Verification items for the finished model (mm, model axes). A direction names the side the tool comes from. Round coordinates to 2 decimals unless told otherwise and drop trailing zeros. Write each loop counter-clockwise with the first axis right and the second up, starting at its lowest first coordinate (ties: lowest second). Pieces come first, ordered by that corner, then holes. Notation, with made-up numbers: M 42.5,1 L 100.5,1 A30 ccw 100.5,36 Z; hole C 81.25,68.25 d9. An arc over 180 degrees is marked long. Answer in a Markdown table with one row per item. Add a question column.
1. Sectioned sample at A-A on x = 0. Record the cut outline in (y, z).
2. Go/stop test with flat-tipped pins: pin 1 Ø3 at (x, y) = (8, 7.64) entering from +Z; pin 2 Ø3 at (y, z) = (-8.5, 5) entering from +X; pin 3 Ø4 at (y, z) = (13, 2) entering from -X; pin 4 Ø2.5 at (x, y) = (0, 17.64) entering from -Z. Record where each tip stops, or that it passes through.
3. Material ranges on probe 1 along Y at (x, z) = (0, 6.75); probe 2 along X at (y, z) = (-2.36, 5); probe 3 along Y at (x, z) = (0, 1.7), recorded low to high.
4. Draft check along Y on faces 5 (the cylindrical face through (-20.724, -22.773, 6.324)), 6 (the cylindrical face through (14.14, -34.4, 0.49)), 7 (the conical face through (23.666, -17.797, 7.618)). Enter one of: pulls with the +Y half, pulls with the -Y half, needs draft (parallel to the pull), parting line crosses it, or undercut.
5. Sectioned sample at C-C on y = -9. Record the cut outline in (x, z), plus the area to 3 significant figures.
6. Sectioned sample at B-B on y = 17.64. Record the cut outline in (x, z), plus the area to 3 significant figures.
7. Set-up check for faces 1 (the flat face through (0, -35, 1)), 2 (the flat face through (-18, -16.5, 4)), 3 (the flat face through (14.5, 2, 4)), 4 (the cylindrical face through (-0.27, -29.43, 2.33)): record each of +Z, -Z, +X, -X, +Y, -Y from which the full face is reachable in a straight line by a thin tool's end or side.
```python
from build123d import *

# Parameters (mm, degrees)
SKETCH1_W                                           = 50
SKETCH1_H                                           = 73
BOSS_EXTRUDE1_DEPTH                                 = 8
CBORE_FOR_M3_HEX_SOCKET_HEAD_CAP_SCREW1_D           = 3.4
CBORE_FOR_M3_HEX_SOCKET_HEAD_CAP_SCREW1_CBORE_D     = 6.5
CBORE_FOR_M3_HEX_SOCKET_HEAD_CAP_SCREW1_CBORE_DEPTH = 3.4
CUT_EXTRUDE1_DEPTH                                  = 3.4
CUT_EXTRUDE2_DEPTH                                  = 16.4
SKETCH9_W                                           = 50
SKETCH9_H                                           = 13
CUT_EXTRUDE3_DEPTH                                  = 10
CUT_EXTRUDE6_DEPTH                                  = 49
FILLET1_R                                           = 3
FILLET2_R                                           = 2
M4_TAPPED_HOLE1_D                                   = 3.3
M4_TAPPED_HOLE1_DEPTH                               = 6
M4_TAPPED_HOLE1_TIP                                 = 0.991420021
CUT_EXTRUDE9_DEPTH                                  = 1
CHAMFER2_SIZE                                       = 1
CHAMFER3_SIZE                                       = 1


with BuildPart() as part:
    # Sketch1 → Boss-Extrude1 (new body)
    with BuildSketch(Plane.XY):
        Rectangle(SKETCH1_W, SKETCH1_H)
    extrude(amount=BOSS_EXTRUDE1_DEPTH)

    # CBORE for M3 Hex Socket Head Cap Screw1 (through all)
    with Locations(Plane.XY.offset(8)):
        with Locations((0, 17.64)):
            CounterBoreHole(CBORE_FOR_M3_HEX_SOCKET_HEAD_CAP_SCREW1_D / 2, CBORE_FOR_M3_HEX_SOCKET_HEAD_CAP_SCREW1_CBORE_D / 2, CBORE_FOR_M3_HEX_SOCKET_HEAD_CAP_SCREW1_CBORE_DEPTH)

    # Sketch5 → Cut-Extrude1 (cut)
    with BuildSketch(Plane.XY.offset(8)):
        with BuildLine():
            ThreePointArc((-19.034141209, -27.101138862), (0, -30.981682799), (19.034141209, -27.101138862))
            ThreePointArc((19.034141209, -27.101138862), (20.752463932, -22.838232925), (16.489557996, -21.119910203))
            ThreePointArc((16.489557996, -21.119910203), (0, -24.481682799), (-16.489557996, -21.119910203))
            ThreePointArc((-16.489557996, -21.119910203), (-20.752463932, -22.838232925), (-19.034141209, -27.101138862))
        make_face()
    extrude(amount=-CUT_EXTRUDE1_DEPTH, mode=Mode.SUBTRACT)

    # Sketch6 → Cut-Extrude2 (cut)
    with BuildSketch(Plane.XY.offset(4.6)):
        with BuildLine():
            ThreePointArc((-18.427355981, -25.674845874), (0, -29.431682799), (18.427355981, -25.674845874))
            ThreePointArc((18.427355981, -25.674845874), (19.326170944, -23.445018153), (17.096343223, -22.546203191))
            ThreePointArc((17.096343223, -22.546203191), (0, -26.031682799), (-17.096343223, -22.546203191))
            ThreePointArc((-17.096343223, -22.546203191), (-19.326170944, -23.445018153), (-18.427355981, -25.674845874))
        make_face()
    extrude(amount=-CUT_EXTRUDE2_DEPTH, mode=Mode.SUBTRACT)

    # Sketch9 → Cut-Extrude3 (cut)
    with BuildSketch(Plane.XY.offset(8)):
        with Locations((0, 30)):
            Rectangle(SKETCH9_W, SKETCH9_H)
    extrude(amount=-CUT_EXTRUDE3_DEPTH, mode=Mode.SUBTRACT)

    # Sketch10 → Cut-Extrude6 (cut)
    with BuildSketch(Plane.XY.offset(8)):
        Polygon((-14.5, 23.5), (-14.5, -16.5), (-25, -16.5), (-32.867212943, -16.5), (-35.349336633, 40.207518582), (-6.106494824, 43.004037027), (18.040764003, 43.004037027), (35.555684922, 29.266712136), (37.966370543, 22.69314443), (41.94143417, 11.853759291), (39.953902356, 3.910005632), (32.212385861, -8.825532839), (28.601359922, -14.76601747), (25, -16.5), (14.5, -16.5), (14.5, 23.5), align=None)
    extrude(amount=-CUT_EXTRUDE6_DEPTH, mode=Mode.SUBTRACT)

    # Fillet1
    fillet1_edges = [part.edges().sort_by_distance(p)[0] for p in [
        (25, -36.5, 4),
        (-25, -36.5, 4),
        (25, -16.5, 4),
        (-25, -16.5, 4),
    ]]
    fillet(fillet1_edges, radius=FILLET1_R)

    # Fillet2
    fillet2_edges = [part.edges().sort_by_distance(p)[0] for p in [
        (-14.5, 23.5, 4),
        (14.5, 23.5, 4),
    ]]
    fillet(fillet2_edges, radius=FILLET2_R)

    # M4 Tapped Hole1
    with Locations(Plane.XY.offset(8)):
        with Locations((-8, -2.36), (8, -2.36), (-8, 7.64), (8, 7.64)):
            Hole(M4_TAPPED_HOLE1_D / 2, depth=M4_TAPPED_HOLE1_DEPTH)
            with Locations((0, 0, -(M4_TAPPED_HOLE1_DEPTH + M4_TAPPED_HOLE1_TIP / 2))):  # 118° drill point
                Cone(0, M4_TAPPED_HOLE1_D / 2, M4_TAPPED_HOLE1_TIP, mode=Mode.SUBTRACT)

    # Sketch14 → Cut-Extrude9 (cut)
    with BuildSketch(Plane(origin=(0, 0, 0), x_dir=(-1, 0, 0), z_dir=(0, 0, -1))):
        with BuildLine():
            Line((-12, -33.5), (12, -33.5))
            ThreePointArc((12, -33.5), (14.121320344, -34.378679656), (15, -36.5))
            Line((15, -36.5), (-15, -36.5))
            ThreePointArc((-15, -36.5), (-14.121320344, -34.378679656), (-12, -33.5))
        make_face()
    extrude(amount=-CUT_EXTRUDE9_DEPTH, mode=Mode.SUBTRACT)

    # Chamfer2
    chamfer2_edges = [part.edges().sort_by_distance(p)[0] for p in [
        (-18.25, -16.5, 8),
        (18.25, -16.5, 8),
        (-24.121320344, -17.378679656, 8),
        (24.121320344, -17.378679656, 8),
        (-25, -26.5, 8),
        (25, -26.5, 8),
        (-24.121320344, -35.621320344, 8),
        (24.121320344, -35.621320344, 8),
        (0, -36.5, 8),
        (-14.5, 2.5, 0),
        (-13.914213562, 22.914213562, 0),
        (0, 23.5, 0),
        (13.914213562, 22.914213562, 0),
        (14.5, 2.5, 0),
        (18.25, -16.5, 0),
        (24.121320344, -17.378679656, 0),
        (25, -26.5, 0),
        (24.121320344, -35.621320344, 0),
        (18.5, -36.5, 0),
        (-18.25, -16.5, 0),
        (-24.121320344, -17.378679656, 0),
        (-25, -26.5, 0),
        (-24.121320344, -35.621320344, 0),
        (-18.5, -36.5, 0),
    ]]
    chamfer(chamfer2_edges, length=CHAMFER2_SIZE)

    # Chamfer3
    chamfer3_edges = [part.edges().sort_by_distance(p)[0] for p in [
        (14.5, 2, 8),
        (13.914213562, 22.914213562, 8),
        (0, 23.5, 8),
        (-13.914213562, 22.914213562, 8),
        (-14.5, 2, 8),
    ]]
    chamfer(chamfer3_edges, length=CHAMFER3_SIZE)


solid = part.part
```
Geometry check:
| question | item | result |
|---|---|---|
| 1 | outline | M -36.5,1 L -33.5,1 L -33.5,0 L -29.43,0 L -29.43,4.6 L -30.98,4.6 L -30.98,8 L -35.5,8 L -36.5,7 Z; M -26.03,0 L 15.94,0 L 15.94,4.6 L 14.39,4.6 L 14.39,8 L -24.48,8 L -24.48,4.6 L -26.03,4.6 Z; M 19.34,0 L 22.5,0 L 23.5,1 L 23.5,7 L 22.5,8 L 20.89,8 L 20.89,4.6 L 19.34,4.6 Z |
| 2 | pin 1 | stops at z = 1.91 |
| 2 | pin 2 | stops at x = 14.5 |
| 2 | pin 3 | stops at x = -14.5 |
| 2 | pin 4 | passes through |
| 3 | probe 1 | y = -36.5 to -30.98, -24.48 to 14.39, 20.89 to 23.5 |
| 3 | probe 2 | x = -14.5 to -9.65, -6.35 to 6.35, 9.65 to 14.5 |
| 3 | probe 3 | y = -36.5 to -29.43, -26.03 to 15.94, 19.34 to 23.5 |
| 4 | face 5 | undercut |
| 4 | face 6 | pulls with the -Y half |
| 4 | face 7 | pulls with the +Y half |
| 5 | outline | M -14.5,1 L -13.5,0 L 13.5,0 L 14.5,1 L 14.5,7 L 13.5,8 L -13.5,8 L -14.5,7 Z |
| 5 | area | 230 mm2 |
| 6 | outline | M -14.5,1 L -13.5,0 L -1.7,0 L -1.7,4.6 L -3.25,4.6 L -3.25,8 L -13.5,8 L -14.5,7 Z; M 1.7,0 L 13.5,0 L 14.5,1 L 14.5,7 L 13.5,8 L 3.25,8 L 3.25,4.6 L 1.7,4.6 Z |
| 6 | area | 192 mm2 |
| 7 | face 1 | -Z, -Y |
| 7 | face 2 | +Z, -Z, -X, +Y |
| 7 | face 3 | +Z, -Z, +X, +Y |
| 7 | face 4 | +Z, -Z |
